Autodesk Inventor part; units mm, degrees
ref_plane "YZ Plane" through (0, 0, 0) normal (1, 0, 0) x (0, 1, 0)
ref_plane "XZ Plane" through (0, 0, 0) normal (0, 1, 0) x (-1, 0, 0)
ref_plane "XY Plane" through (0, 0, 0) normal (0, 0, 1) x (1, 0, 0)
sketch "Sketch1" plane through (0, 0, 0) normal (0, 0, 1) x (1, 0, 0)
  line L0 (-651.5983, 84.4921) -> (440.9045, 84.4921)
  line L1 (440.9045, 84.4921) -> (440.9045, -15.5079)
  line L2 (440.9045, -15.5079) -> (-651.5983, -15.5079)
  line L3 (-651.5983, -15.5079) -> (-651.5983, 84.4921)
  line L4 (-651.5983, -15.5079) -> (-899.2765, -81.873)
  point P0 (0, 0)
  dimension "d0" = 100
extrude "Extrusion1" add sketch "Sketch1" against normal blind 60
fillet "Fillet1" radius 3 4 edges at (-105.3469, 84.4921, 0) (-105.3469, 84.4921, -60) (-105.3469, -15.5079, 0) (-105.3469, -15.5079, -60)
shell "Shell1" thickness 3 removed faces 2 at (440.9045, 18.8255, -40) at (-651.5983, 18.8255, -40)
sketch "Sketch2" plane through (0, 0, 0) normal (0, 0, 1) x (1, 0, 0)
  circle A0 centre (377.8245, 22.8431) radius 11.25
  point P0 (0, 0)
extrude "Extrusion2" cut sketch "Sketch2" against normal through all
sketch "Sketch3" plane through (-651.5983, 84.4921, -57) normal (0, 1, 0) x (1, 0, 0)
  line L0 (0, 0) -> (1092.5029, 0)
  line L1 (0, -54) -> (0, 0)
  line L2 (1092.5029, -54) -> (0, -54)
  line L3 (1092.5029, -54) -> (1092.5029, 0)
  line L4 (1092.5029, -54) -> (998.9721, 0)
  line L5 (0, 0) -> (1092.5029, 0)
  line L6 (1092.5029, -54) -> (1101.6667, -54)
  line L7 (1101.6667, -54) -> (1101.6667, 18.4263)
  line L8 (1101.6667, 18.4263) -> (998.9721, 18.4263)
  line L9 (998.9721, 18.4263) -> (998.9721, 0)
  point P0 (651.5983, -57)
  dimension "d8" = 30
extrude "Extrusion3" cut sketch "Sketch3" against normal through all contours L9 L8 L7 L6 L3 L0 | L0 L3 L4
properties part number "Barra nuevo pivote"
Geometry check sheet. Reference: the model listing, model coordinates, mm. A direction names the side the tool comes from. Give positions to 0.01 mm unless a question says otherwise; leave off trailing zeros. Write each loop counter-clockwise with the first axis right and the second up, starting at its lowest first coordinate (ties: lowest second). Pieces come first, ordered by that corner, then holes. Notation, with made-up numbers: (13, 27.5) - (55, 27.5) arc R21 cw to (55, 48.5) - close; hole circle Ø7 at (20, 62.5). An arc over 180 degrees is marked (long way). Put each result on its own line as item: value.
1. Sectioned sample at C-C, the plane x = -378. Enter the section's corners in (y, z).
Ans:
outline: (-15.51, -57) arc R3 ccw to (-12.51, -60) - (81.49, -60) arc R3 ccw to (84.49, -57) - (84.49, -3) arc R3 ccw to (81.49, 0) - (-12.51, 0) arc R3 ccw to (-15.51, -3) - close; hole (-12.51, -57) - (81.49, -57) - (81.49, -3) - (-12.51, -3) - close
2. Set-up check for faces 1 (the flat face through (-113, 35, 0)), 2 (the flat face through (-113, 81.492, -30)): record each of +Z, -Z, +X, -X, +Y, -Y from which the full face is reachable in a straight line by a thin tool's end or side.
Ans:
face 1: +Z, +X, -X, +Y, -Y
face 2: +X, -X
3. Sectioned sample at B-B, the plane z = -43. Enter the section's corners in (x, y).
Ans:
outline: (-651.6, -15.51) - (371.62, -15.51) - (371.62, -12.51) - (-651.6, -12.51) - close; (-651.6, 81.49) - (371.62, 81.49) - (371.62, 84.49) - (-651.6, 84.49) - close
4. Thickness scan on line 1 (Y direction, x = 296, z = -50); line 2 (Z direction, x = 231, y = 27); line 3 (Z direction, x = 355.5, y = 33). Record the ranges inside material, lowest first.
Ans:
line 1: y = -15.51 to -12.51, 81.49 to 84.49
line 2: z = -60 to -57, -3 to 0
line 3: z = -3 to 0
5. Draft check along Y on faces 3 (the flat face through (-98, -12.508, -30)), 4 (the flat face through (-98, -15.508, -30)), 5 (the flat face through (394.794, 83.013, -29.622)). Enter one of: +Y half, -Y half, draft (parallel to the pull), parting line (faces both ways), or undercut.
Ans:
face 3: undercut
face 4: -Y half
face 5: draft
6. Go/stop test with a flat-tipped pin: pin 1 (2.5 mm diameter, centred on y = 59, z = -59, fed in from +X). Record where the tip stops, or that it passes through.
Ans:
pin 1: stops at x = 347.37
7. Sectioned sample at A-A, the plane y = 70.5. Enter the section's corners in (x, z).
Ans:
outline: (-651.6, -60) - (347.37, -60) - (347.37, -57) - (-651.6, -57) - close; (-651.6, -3) - (440.9, -3) - (440.9, 0) - (-651.6, 0) - close
